from build123d import *

# Parameters (mm, degrees)
BOSS_EXTRUDE1_DEPTH      = 1.5875
BOSS_EXTRUDE1_DEPTH_BACK = 1.5875
SKETCH1_W                = 600
SKETCH1_H                = 600
SKETCH1_R                = 3.25
SKETCH1_R_2              = 150
SKETCH3_R                = 4.1
CUT_EXTRUDE2_DEPTH       = 425.267038734
CIRPATTERN1_COUNT        = 4


with BuildPart() as part:
    # Sketch1 → Boss-Extrude1 (new, two sides: drawn at the far end of the back side and taken through both)
    with BuildSketch(Plane(origin=(0, 0, 0), x_dir=(1, 0, 0), z_dir=(0, 1, 0)).offset(-BOSS_EXTRUDE1_DEPTH_BACK)):
        Rectangle(SKETCH1_W, SKETCH1_H)
        with Locations(Location((125, 250, 0), (0, 0, 270))):
            Circle(SKETCH1_R, mode=Mode.SUBTRACT)
        with Locations(Location((-125, -250, 0), (0, 0, 270))):
            Circle(SKETCH1_R, mode=Mode.SUBTRACT)
        with Locations(Location((0, 0, 0), (0, 0, 270))):
            Circle(SKETCH1_R_2, mode=Mode.SUBTRACT)
    extrude(amount=BOSS_EXTRUDE1_DEPTH + BOSS_EXTRUDE1_DEPTH_BACK)

    # Sketch3 → Cut-Extrude2 (cut, symmetric)
    with BuildSketch(Plane(origin=(0, 0, 0), x_dir=(1, 0, 0), z_dir=(0, 1, 0))):
        with Locations(Location((0, 280, 0), (0, 0, 270))):
            Circle(SKETCH3_R)
        with Locations(Location((-120, 280, 0), (0, 0, 270))):
            Circle(SKETCH3_R)
        with Locations(Location((-240, 280, 0), (0, 0, 270))):
            Circle(SKETCH3_R)
        with Locations(Location((240, 280, 0), (0, 0, 90))):
            Circle(SKETCH3_R)
        with Locations(Location((120, 280, 0), (0, 0, 90))):
            Circle(SKETCH3_R)
    cut_extrude2 = extrude(amount=CUT_EXTRUDE2_DEPTH, both=True, mode=Mode.SUBTRACT)

    # CirPattern1: Cut-Extrude2 ×4 about axis
    cirpattern1_axis = Axis((0, 0, 0), (0, 1, 0))
    for i in range(1, CIRPATTERN1_COUNT):
        add(cut_extrude2.rotate(cirpattern1_axis, i * 360 / CIRPATTERN1_COUNT), mode=Mode.SUBTRACT)


solid = part.part
For this review, take the finished solid that the model builds, in its own axes (mm). Round coordinates to 2 decimals unless told otherwise and drop trailing zeros. Loops run counter-clockwise (first coordinate to the right, second up) from the corner with the lowest first, then second, coordinate; pieces in that order, holes last. Notation, with made-up numbers: (68, 81) - (79, 81) arc R25 ccw to (79, 110) - close; hole circle Ø3 at (15.5, 13). An arc over 180 degrees is marked (long way). Put each result on its own line as item: value. Start each with the question number.
1. Consider section C-C on z = -75. State the section outline as (x, y) points.
2. Insertion check: P1, Ø7.5, axis at x = -280, z = 0, coming from the -Y side. The pin has a flat end and moves straight along its axis. Give the tip position at first contact, or say it passes through.
3. For probe 1 along X at (y, z) = (-0.05, 280); probe 2 along X at (y, z) = (1.2, 239), list the stretches that pass through material, from the lowest coordinate up. Write a range as [from, to].
4. Consider section B-B on z = -138. State the section outline as (x, y) points.
5. Mouldability with a two-part tool opening along X and no side actions: class faces 1 (the flat face through (-138, 1.588, -71)), 2 (the cylindrical face through (-91.273, -0.022, -119.035)) as +X half, -X half, draft (parallel to the pull), parting line (faces both ways), or undercut.
6. Consider section A-A on y = -0.95. State how many separate pieces and enclosed holes the cut face has, plus the area to 3 significant figures.
Result sheet:
1. outline: (-300, -1.59) - (-129.9, -1.59) - (-129.9, 1.59) - (-300, 1.59) - close; (129.9, -1.59) - (300, -1.59) - (300, 1.59) - (129.9, 1.59) - close
2. P1: through
3. probe 1: [-300, -244.1], [-235.9, -124.1], [-115.9, -4.1], [4.1, 115.9], [124.1, 235.9], [244.1, 300]
3. probe 2: [-300, -283.98], [-276.02, 276.02], [283.98, 300]
4. outline: (-300, -1.59) - (-58.79, -1.59) - (-58.79, 1.59) - (-300, 1.59) - close; (58.79, -1.59) - (300, -1.59) - (300, 1.59) - (58.79, 1.59) - close
5. face 1: draft
5. face 2: undercut
6. separate pieces: 1
6. enclosed holes: 23
6. area: 288,000 mm^2
